Could you check a few things on this model? Use its own coordinates, in mm. A direction names the side the tool comes from. Round coordinates to 2 decimals unless told otherwise and drop trailing zeros. Loops run counter-clockwise (first coordinate to the right, second up) from the corner with the lowest first, then second, coordinate; pieces in that order, holes last. Notation, with made-up numbers: (62.5, -19.75) -> (98.5, -19.75) arc R26 ccw to (98.5, 19.25) -> close; hole circle Ø7 at (61, 43). An arc over 180 degrees is marked (long way). One line per item, written item: value.
```python
from build123d import *

# Parameters (mm, degrees)
SKETCH1_W           = 17
SKETCH1_H           = 20
BOSS_EXTRUDE1_DEPTH = 20
SHELL1_T            = -3
CUT_EXTRUDE1_DEPTH  = 18
CUT_EXTRUDE2_DEPTH  = 4
CUT_EXTRUDE3_DEPTH  = 4


with BuildPart() as part:
    # Sketch1 → Boss-Extrude1 (new body)
    with BuildSketch(Plane(origin=(0, 0, 0), x_dir=(1, 0, 0), z_dir=(0, 1, 0))):
        Rectangle(SKETCH1_W, SKETCH1_H)
    extrude(amount=BOSS_EXTRUDE1_DEPTH)

    # Shell1
    shell1_openings = [part.faces().sort_by_distance(p)[0] for p in [
        (0, 20, 0),
    ]]
    offset(amount=SHELL1_T, openings=shell1_openings, kind=Kind.INTERSECTION)

    # Sketch3 → Cut-Extrude1 (cut, through all)
    with BuildSketch(Plane(origin=(8.5, 0, 0), x_dir=(0, 0, -1), z_dir=(1, 0, 0))):
        Polygon((7, 20), (-10, 20), (-10, 3), align=None)
    extrude(amount=-CUT_EXTRUDE1_DEPTH, mode=Mode.SUBTRACT)

    # Sketch4 → Cut-Extrude2 (cut, through all)
    with BuildSketch(Plane(origin=(0, 3, 0), x_dir=(1, 0, 0), z_dir=(0, 1, 0))):
        with BuildLine():
            Line((1.3, 1.5), (1.3, -1.5))
            ThreePointArc((1.3, -1.5), (0, -2.8), (-1.3, -1.5))
            Line((-1.3, -1.5), (-1.3, 1.5))
            ThreePointArc((-1.3, 1.5), (0, 2.8), (1.3, 1.5))
        make_face()
    extrude(amount=-CUT_EXTRUDE2_DEPTH, mode=Mode.SUBTRACT)

    # Sketch5 → Cut-Extrude3 (cut, through all)
    with BuildSketch(Plane.XY.offset(-7)):
        with BuildLine():
            Line((1.3, 14.5), (1.3, 11.5))
            ThreePointArc((1.3, 11.5), (0, 10.2), (-1.3, 11.5))
            Line((-1.3, 11.5), (-1.3, 14.5))
            ThreePointArc((-1.3, 14.5), (0, 15.8), (1.3, 14.5))
        make_face()
    extrude(amount=-CUT_EXTRUDE3_DEPTH, mode=Mode.SUBTRACT)


solid = part.part
```
Item 1: If we section it at B-B on z = -1: List the corners of the cut face in (x, y) for me.
Output:
outline: (-8.5, 0) -> (-1.3, 0) -> (-1.3, 3) -> (-5.5, 3) -> (-5.5, 14) -> (-8.5, 14) -> close; (1.3, 0) -> (8.5, 0) -> (8.5, 14) -> (5.5, 14) -> (5.5, 3) -> (1.3, 3) -> close
Item 2: For faces 1 (the face through (0, 15.8, -8.5)), 2 (the face through (0, 4, 7)), 3 (the face through (1.3, 2, 0)), which set-ups out of +Z, -Z, +X, -X, +Y, -Y let a thin tool reach every point of the face, with its end or its side?
Output:
face 1: +Z, -Z
face 2: +Y
face 3: +Y, -Y
Item 3: Will these pins go through, and if not, where does the flat tip stop? pin 1 Ø5 at (y, z) = (13, 6.5) entering from -X; pin 2 Ø5.5 at (x, y) = (-0.5, 13) entering from +Z; pin 3 Ø3.5 at (x, z) = (2.5, 0.5) entering from +Y.
Output:
pin 1: passes through
pin 2: stops at z = -7
pin 3: stops at y = 3
Item 4: If we section it at D-D on y = 7: List the corners of the cut face in (x, z) for me.
Output:
outline: (-8.5, -10) -> (8.5, -10) -> (8.5, 6) -> (5.5, 6) -> (5.5, -7) -> (-5.5, -7) -> (-5.5, 6) -> (-8.5, 6) -> close
Item 5: If we section it at A-A on x = 0: List the corners of the cut face in (y, z) for me.
Output:
outline: (0, -10) -> (10.2, -10) -> (10.2, -7) -> (3, -7) -> (3, -2.8) -> (0, -2.8) -> close; (0, 2.8) -> (3, 2.8) -> (3, 7) -> (6, 7) -> (3, 10) -> (0, 10) -> close; (15.8, -10) -> (20, -10) -> (20, -7) -> (15.8, -7) -> close
Item 6: If we section it at C-C on y = 11: List the corners of the cut face in (x, z) for me.
Output:
outline: (-8.5, -10) -> (-1.2, -10) -> (-1.2, -7) -> (-5.5, -7) -> (-5.5, 2) -> (-8.5, 2) -> close; (1.2, -10) -> (8.5, -10) -> (8.5, 2) -> (5.5, 2) -> (5.5, -7) -> (1.2, -7) -> close
Item 7: If we mould it in two halves opening along Y, with no side actions, what happens to faces 4 (the face through (-1.3, 13, -8)), 5 (the face through (-1.3, 2, 0)), 6 (the face through (0, 10.2, -8.5)), 7 (the face through (6, 9, 4))? For each: released by +Y, released by -Y, zero draft, split by the parting line, or undercut.
Output:
face 4: undercut
face 5: zero draft
face 6: undercut
face 7: released by +Y
Item 8: I need wall thicknesses on line 1 (Z direction, x = -2.75, y = 4.5); line 2 (Y direction, x = 0, z = 6.25); line 3 (Z direction, x = 4.5, y = 9.75). Which ranges of each line are inside material? Lowest first, please. Write a range as from..to.
Output:
line 1: z = -10..-7, 7..8.5
line 2: y = 0..3
line 3: z = -10..-7
